from build123d import *

# Parameters (mm, degrees)
SKETCH_1_W          = 113
SKETCH_1_H          = 150
SKETCH_1_R          = 2
SKETCH_1_W_2        = 72.084054685
SKETCH_1_H_2        = 108.126082027
EXTRUDE_1_DEPTH     = 10
SKETCH_2_W          = 30
SKETCH_2_H          = 150
EXTRUDE_2_DEPTH     = 12
SKETCH_3_R          = 2.5
CUT_EXTRUDE_2_DEPTH = 12
SKETCH_6_R          = 4.5
CUT_EXTRUDE_5_DEPTH = 5


with BuildPart() as part:
    # 草图1 → 凸台-拉伸1 (new body)
    with BuildSketch(Plane.XY):
        with Locations((36.884615385, -26.807692308)):
            Rectangle(SKETCH_1_W, SKETCH_1_H)
        with Locations((78.884615385, 36.192307692)):
            Circle(SKETCH_1_R, mode=Mode.SUBTRACT)
        with Locations((-5.115384615, 36.192307692)):
            Circle(SKETCH_1_R, mode=Mode.SUBTRACT)
        with Locations((78.884615385, -89.807692308)):
            Circle(SKETCH_1_R, mode=Mode.SUBTRACT)
        with Locations((-5.115384615, -89.807692308)):
            Circle(SKETCH_1_R, mode=Mode.SUBTRACT)
        with Locations((36.884615385, -26.807692307)):
            Rectangle(SKETCH_1_W_2, SKETCH_1_H_2, mode=Mode.SUBTRACT)
    extrude(amount=EXTRUDE_1_DEPTH)

    # 草图2 → 凸台-拉伸2 (add)
    with BuildSketch(Plane(origin=(93.384615385, 0, 0), x_dir=(0, 0, -1), z_dir=(1, 0, 0))):
        with Locations((-15, -26.807692308)):
            Rectangle(SKETCH_2_W, SKETCH_2_H)
    extrude(amount=EXTRUDE_2_DEPTH)

    # 草图3 → 切除-拉伸2 (cut)
    with BuildSketch(Plane.ZY.offset(-93.384615385)):
        with Locations(Location((20, 38.192307692, 0), (0, 0, 270))):
            Circle(SKETCH_3_R)
        with Locations(Location((20, -91.807692308, 0), (0, 0, 90))):
            Circle(SKETCH_3_R)
    extrude(amount=-CUT_EXTRUDE_2_DEPTH, mode=Mode.SUBTRACT)

    # 草图6 → 切除-拉伸5 (cut)
    with BuildSketch(Plane.ZY.offset(-93.384615385)):
        with Locations(Location((20, 38.192307692, 0), (0, 0, 270))):
            Circle(SKETCH_6_R)
        with Locations(Location((20, -91.807692308, 0), (0, 0, 90))):
            Circle(SKETCH_6_R)
    extrude(amount=-CUT_EXTRUDE_5_DEPTH, mode=Mode.SUBTRACT)


solid = part.part
Here's how the part is built. I have some questions about the finished solid (model axes, mm). A direction names the side the tool comes from. Round coordinates to 2 decimals unless told otherwise and drop trailing zeros. Order: outer loops, then holes, each group sorted by start corner. A loop starts at its lowest first (then second) coordinate and runs counter-clockwise, first axis right, second up. Notation, with made-up numbers: M 45.5,-23.5 L 55.5,-23.5 A13 ccw 55.5,-5.5 Z; hole C 59.25,69 d3. An arc over 180 degrees is marked long. One line per question, with ' | ' between items.
1) Imagine slicing it at B-B, the plane z = 20. Write out the boundary of the cut face in (x, y).
Checked values:
outline: M 93.38,-101.81 L 105.38,-101.81 L 105.38,-94.31 L 98.38,-94.31 L 98.38,-96.31 L 93.38,-96.31 Z; M 93.38,-87.31 L 98.38,-87.31 L 98.38,-89.31 L 105.38,-89.31 L 105.38,35.69 L 98.38,35.69 L 98.38,33.69 L 93.38,33.69 Z; M 93.38,42.69 L 98.38,42.69 L 98.38,40.69 L 105.38,40.69 L 105.38,48.19 L 93.38,48.19 Z
2) Imagine slicing it at C-C, the plane x = 38. Write out the boundary of the cut face in (y, z), plus the area to 3 significant figures.
Checked values:
outline: M -101.81,0 L -80.87,0 L -80.87,10 L -101.81,10 Z; M 27.26,0 L 48.19,0 L 48.19,10 L 27.26,10 Z | area: 419 mm²
3) We'd pull the mould along Y, two halves only. Please class faces 4 (the flat face through (98.385, 36, 18)), 5 (the flat face through (56, -101.808, 9)), 6 (the flat face through (93.385, -26, 20)): released by +Y, released by -Y, zero draft, split by the parting line, or undercut.
Checked values:
face 4: undercut | face 5: released by -Y | face 6: zero draft
4) Imagine slicing it at A-A, the plane y = -27. Write out the boundary of the cut face in (x, z), plus the area to 3 significant figures.
Checked values:
outline: M -19.62,0 L 0.84,0 L 0.84,10 L -19.62,10 Z; M 72.93,0 L 105.38,0 L 105.38,30 L 93.38,30 L 93.38,10 L 72.93,10 Z | area: 769 mm²
5) I'm going to push flat-ended pins straight in: pin 1 Ø12 at (y, z) = (-65.5, 25.5) entering from -X; pin 2 Ø6 at (x, y) = (79.5, -2.5) entering from +Z. Where does each tip first touch, or does it pass through?
Checked values:
pin 1: stops at x = 93.38 | pin 2: stops at z = 10
6) I need wall thicknesses on line 1 (X direction, y = 4, z = 9.25); line 2 (Y direction, x = -6, z = 9); line 3 (Y direction, x = 52, z = 7). Which ranges of each line are inside material? Lowest first, please.
Checked values:
line 1: x = -19.62 to 0.84, 72.93 to 105.38 | line 2: y = -101.81 to -91.6, -88.01 to 34.4, 37.99 to 48.19 | line 3: y = -101.81 to -80.87, 27.26 to 48.19
7) Imagine slicing it at D-D, the plane z = 2.25. Write out the boundary of the cut face in (x, y), plus the area to 3 significant figures.
Checked values:
outline: M -19.62,-101.81 L 105.38,-101.81 L 105.38,48.19 L -19.62,48.19 Z; hole C -5.12,-89.81 d4; hole C -5.12,36.19 d4; hole M 0.84,-80.87 L 72.93,-80.87 L 72.93,27.26 L 0.84,27.26 Z; hole C 78.88,-89.81 d4; hole C 78.88,36.19 d4 | area: 10,900 mm²
8) On a 3-axis mill with a long thin cutter (end or side, diameter ignored), from which of +Z, -Z, +X, -X, +Y, -Y can I reach the whole of each face in a straight line? I mean faces 1 (the flat face through (-2, -26, 10)), 2 (the flat face through (98.385, -90, 22)), 3 (the flat face through (36, -80.871, 5)). Say none if no direction works.
Checked values:
face 1: +Z, -X, +Y, -Y | face 2: -X | face 3: +Z, -Z
